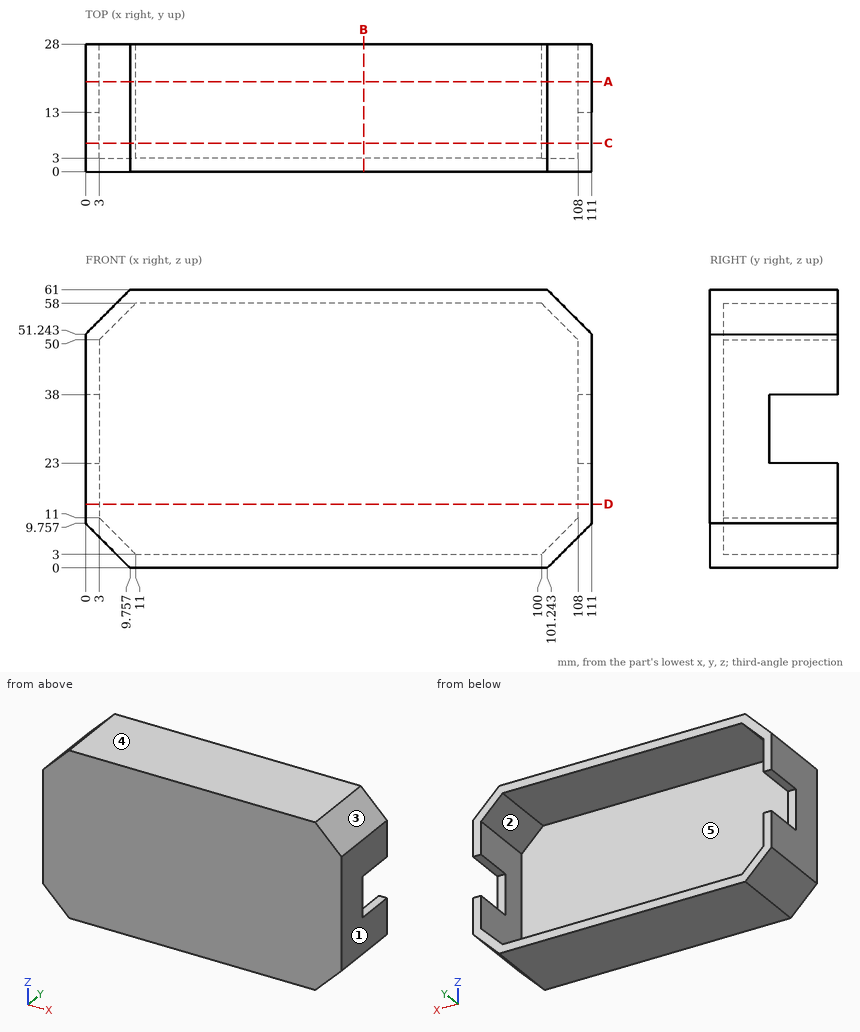
The figure shows three views and two pictorial views of one solid part (mm, origin at its lowest corner). Answer the questions. A direction names the side the tool comes from. Coordinates: 2 decimals unless noted, no trailing zeros. Loops run counter-clockwise (first coordinate to the right, second up) from the corner with the lowest first, then second, coordinate; pieces in that order, holes last.
1) Find section C-C on y = 6.25. Write down the section's boundary in (x, z).
2) Find section D-D on z = 14. Write down the section's boundary in (x, y).
3) Determine the mould class of the marked faces 3, 4 and 5 for opening direction X: pulls with the +X half, pulls with the -X half, needs draft (parallel to the pull), parting line crosses it, or undercut.
4) Find the intervals of material crossed by L1, parallel to Z at x = 86, y = 11.25; L2, parallel to X at y = 8.5, z = 44; L3, parallel to Y at x = 82, z = 55, in increasing order.
5) Find section B-B on x = 61. Write down the section's boundary in (y, z).
6) Flat-ended cylindrical pins translate along their axes: pin 1 Ø4 at (y, z) = (18.5, 25.5) entering from -X; pin 2 Ø1.5 at (x, y) = (109.5, 21.5) entering from -Z; pin 3 Ø1.5 at (x, z) = (109.5, 27.5) entering from +Y; pin 4 Ø5 at (y, z) = (15, 9.5) entering from +X. Find the tip coordinate at first contact, or state that the pin passes through.
7) Find section A-A on y = 19.75. Write down the section's boundary in (x, z).
8) A tool of negligible diameter and unlimited length cuts with its end or side. For the marked faces 1 and 2, from which of +Z, -Z, +X, -X, +Y, -Y can it reach the whole face along a straight path? Write none if from no direction.
Values:
1. outline: (0, 9.76) - (9.76, 0) - (101.24, 0) - (111, 9.76) - (111, 51.24) - (101.24, 61) - (9.76, 61) - (0, 51.24) - close; hole (3, 11) - (11, 3) - (100, 3) - (108, 11) - (108, 50) - (100, 58) - (11, 58) - (3, 50) - close
2. outline: (0, 0) - (111, 0) - (111, 28) - (108, 28) - (108, 3) - (3, 3) - (3, 28) - (0, 28) - close
3. face 3: pulls with the +X half
3. face 4: needs draft
3. face 5: undercut
4. L1: z = 0 to 3, 58 to 61
4. L2: x = 0 to 3, 108 to 111
4. L3: y = 0 to 3
5. outline: (0, 0) - (28, 0) - (28, 3) - (3, 3) - (3, 58) - (28, 58) - (28, 61) - (0, 61) - close
6. pin 1: passes through
6. pin 2: stops at z = 7.51
6. pin 3: stops at y = 13
6. pin 4: stops at x = 111
7. outline: (0, 9.76) - (9.76, 0) - (101.24, 0) - (111, 9.76) - (111, 23) - (108, 23) - (108, 11) - (100, 3) - (11, 3) - (3, 11) - (3, 23) - (0, 23) - close; (0, 38) - (3, 38) - (3, 50) - (11, 58) - (100, 58) - (108, 50) - (108, 38) - (111, 38) - (111, 51.24) - (101.24, 61) - (9.76, 61) - (0, 51.24) - close
8. face 1: +Z, -Z, +X, +Y, -Y
8. face 2: +Y
